Check sheet for the modelled part. Datum: model origin and axes. Units: mm. Face numbers are marked on the shaded views. A direction names the side the tool comes from. Round coordinates to 2 decimals unless told otherwise and drop trailing zeros. Loops run counter-clockwise (first coordinate to the right, second up) from the corner with the lowest first, then second, coordinate; pieces in that order, holes last. Notation, with made-up numbers: (-22, 64.25) - (-2, 64.25) arc R23 cw to (-2, 82.25) - close; hole circle Ø9 at (17.5, -17). An arc over 180 degrees is marked (long way). Put each result on its own line as item: value. Start each with the question number.
Item 1: Section check D-D, the plane z = -20.5. Record the cut outline in (x, y) (1 decimal).
Item 2: Section check B-B, the plane x = 20.5. Record the cut outline in (y, z), and give its area (3 significant figures).
Item 3: Section check A-A, the plane z = -38. Record the cut outline in (x, y) (1 decimal).
Item 4: Gauge pin test, flat ends, axial feed: pin 1 Ø5 at (x, y) = (-21.5, 1.5) entering from -Z; pin 2 Ø3 at (x, y) = (21.5, 108) entering from +Z; pin 3 Ø12 at (x, z) = (-7, 0) entering from +Y. Record the tip position at first contact, or that the pin passes through.
Item 5: Draft check along Y on the marked faces 1, 2 and 3. Enter one of: pulls with the +Y half, pulls with the -Y half, needs draft (parallel to the pull), parting line crosses it, or undercut.
Item 6: Section check C-C, the plane y = 17. Record the cut outline in (x, z) (3 decimals).
Item 7: Tool access check on the marked faces 4, 5 and 6. Record the directions out of +Z, -Z, +X, -X, +Y, -Y that give a thin tool (end or side, any length) a straight path to the whole face; none if there is none.
Item 8: Material ranges on line 1 along Z through (x, y) = (21.5, 38); line 2 along Y through (x, z) = (12, -8); line 3 along Z through (x, y) = (2, -13), recorded low to high.
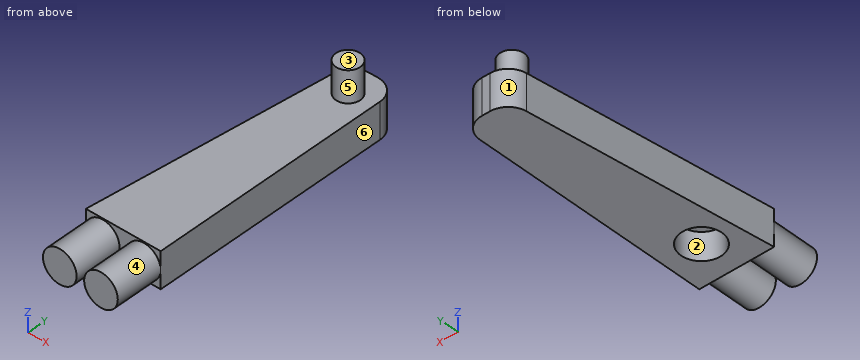
Autodesk Inventor part; units mm, degrees
ref_plane "YZ Plane" through (0, 0, 0) normal (1, 0, 0) x (0, 1, 0)
ref_plane "XZ Plane" through (0, 0, 0) normal (0, 1, 0) x (-1, 0, 0)
ref_plane "XY Plane" through (0, 0, 0) normal (0, 0, 1) x (1, 0, 0)
sketch "Sketch1" plane through (0, 0, 0) normal (0, 0, 1) x (1, 0, 0)
  circle A0 centre (0, 0) radius 30.734
  line L0 (-56.515, -58.42) -> (56.515, -58.42)
  line L1 (56.515, -58.42) -> (56.515, 335.28)
  line L2 (56.515, 335.28) -> (-13.335, 335.28)
  line L3 (-13.335, 335.28) -> (-56.515, -58.42)
  dimension "d0" = 61.468
  dimension "d1" = 393.7
  dimension "d2" = 113.03
  dimension "d3" = 69.85
  dimension "d4" = 58.42
  dimension "d5" = 56.515
extrude "Extrusion1" add sketch "Sketch1" against normal blind 54.3243
fillet "Fillet1" radius 30.48 2 edges at (56.515, 335.28, -27.1621) (-13.335, 335.28, -27.1621)
sketch "Sketch2" plane through (-56.515, -58.42, 0) normal (0, -1, 0) x (1, 0, 0)
  line L0 (113.03, 0) -> (113.03, -54.3243)
  line L1 (113.03, -27.1621) -> (0, -27.1621)
  line L2 (0, 0) -> (0, -54.3243)
  line L3 (56.515, -27.1621) -> (56.515, -44.3071)
  circle A0 centre (87.63, -27.1621) radius 25.4
  circle A1 centre (25.4, -27.1621) radius 25.4
  point P0 (56.515, 0)
  dimension "d10" = 50.8
  dimension "d9" = 50.8
  dimension "d11" = 113.03
extrude "Extrusion2" add sketch "Sketch2" along normal blind 71.12
sketch "Sketch3" plane through (0, 0, 0) normal (0, 0, 1) x (1, 0, 0)
  circle A0 centre (0, 0) radius 42.7153
extrude "Extrusion3" add sketch "Sketch3" against normal blind 12.7
sketch "Sketch4" plane through (0, 0, -54.3243) normal (0, 0, -1) x (-1, 0, 0)
  line L0 (-26.035, 335.28) -> (-13.9848, 335.28)
  line L1 (-20.0099, 335.28) -> (-20.0099, 292.1)
  circle A0 centre (-20.0099, 292.1) radius 18.415
  point P0 (0, 0)
  dimension "d17" = 36.83
  dimension "d20" = 292.1
extrude "Extrusion4" add sketch "Sketch4" against normal blind 101.6
equation "\"d10\" = d9"
properties part number "Forearm-lrg"
Check result:
1. outline: (-56.5, -58.4) - (-55.6, -58.4) - (-55.6, -129.5) - (-6.6, -129.5) - (-6.6, -58.4) - (6.6, -58.4) - (6.6, -129.5) - (55.6, -129.5) - (55.6, -58.4) - (56.5, -58.4) - (56.5, 304.8) arc R30.5 ccw to (26, 335.3) - (14, 335.3) arc R30.5 ccw to (-16.3, 308.1) - close; hole circle Ø61.5 at (0, 0)
2. outline: (-129.54, -50.24) - (-58.42, -50.24) - (-58.42, -54.32) - (-22.9, -54.32) - (-22.9, -12.7) - (22.9, -12.7) - (22.9, -54.32) - (335.28, -54.32) - (335.28, 0) - (310.51, 0) - (310.51, 47.28) - (273.69, 47.28) - (273.69, 0) - (-58.42, 0) - (-58.42, -4.09) - (-129.54, -4.09) - close
2. area: 24,500 mm²
3. outline: (-56.5, -58.4) - (-54.1, -58.4) - (-54.1, -129.5) - (-8.1, -129.5) - (-8.1, -58.4) - (8.1, -58.4) - (8.1, -129.5) - (54.1, -129.5) - (54.1, -58.4) - (56.5, -58.4) - (56.5, 304.8) arc R30.5 ccw to (26, 335.3) - (14, 335.3) arc R30.5 ccw to (-16.3, 308.1) - close; hole circle Ø61.5 at (0, 0)
4. pin 1: z = -12.7
4. pin 2: z = 0
4. pin 3: y = 331.34
5. face 1: pulls with the +Y half
5. face 2: undercut
5. face 3: needs draft
6. outline: (-48.243, -54.324) - (-25.604, -54.324) - (-25.604, -12.7) - (25.604, -12.7) - (25.604, -54.324) - (56.515, -54.324) - (56.515, 0) - (-48.243, 0) - close
7. face 4: -Y
7. face 5: +Z
7. face 6: +Z, -Z, +X, +Y, -Y
8. line 1: -54.32 to 0
8. line 2: -58.42 to 335.22
8. line 3: -12.7 to 0
